Autodesk Inventor part; units mm, degrees
ref_plane "YZ Plane" through (0, 0, 0) normal (1, 0, 0) x (0, 1, 0)
ref_plane "XZ Plane" through (0, 0, 0) normal (0, 1, 0) x (-1, 0, 0)
ref_plane "XY Plane" through (0, 0, 0) normal (0, 0, 1) x (1, 0, 0)
sketch "Sketch1" plane through (0, 0, 0) normal (0, 0, 1) x (1, 0, 0)
  arc A0 (-39.344, -1.4316) -> (39.344, -1.4316) centre (0, 0) ccw
  line L0 (-39.344, -1.4316) -> (-39.3671, -1.4316)
  line L1 (-39.344, -1.4316) -> (-52.044, -1.4316)
  line L2 (39.344, -1.4316) -> (52.044, -1.4316)
  arc A1 (-46.964, -22.4724) -> (46.964, -22.4724) centre (0, 0) ccw
  line L3 (0, -52.0636) -> (0, -55.2386)
  line L4 (0, -55.2386) -> (-72.364, -55.2386)
  line L5 (0, -55.2386) -> (72.364, -55.2386)
  line L6 (-52.044, -1.4316) -> (-59.664, -1.4316)
  line L7 (52.044, -1.4316) -> (59.664, -1.4316)
  line L8 (39.344, -1.4316) -> (46.964, -1.4316)
  line L9 (46.964, -1.4316) -> (46.964, -22.4724)
  line L10 (-39.344, -1.4316) -> (-45.694, -1.4316)
  line L11 (-39.344, -1.4316) -> (-46.964, -1.4316)
  line L12 (-46.964, -1.4316) -> (-46.964, -22.4724)
  line L13 (-46.964, -7.7816) -> (-59.664, -7.7816)
  line L14 (-59.664, -7.7816) -> (-59.664, -1.4316)
  line L15 (46.964, -7.7816) -> (59.664, -7.7816)
  line L16 (59.664, -7.7816) -> (59.664, -1.4316)
  line L17 (-72.364, -55.2386) -> (-72.364, -42.5386)
  line L18 (72.364, -55.2386) -> (72.364, -42.5386)
  line L19 (-72.364, -42.5386) -> (-30.0181, -42.5386)
  line L20 (72.364, -42.5386) -> (30.0181, -42.5386)
  dimension "d0" = 78.74
  dimension "d2" = 12.7
  dimension "d3" = 12.7
  dimension "d4" = 3.175
  dimension "d5" = 7.62
  dimension "d6" = 7.62
  dimension "d7" = 7.62
  dimension "d9" = 7.62
  dimension "d10" = 6.35
  dimension "d11" = 6.35
  dimension "d14" = 12.7
  dimension "d15" = 12.7
extrude "Extrusion1" add sketch "Sketch1" along normal blind 12.7
fillet "Fillet1" radius 7.62 2 edges at (30.0181, -42.5386, 6.35) (-30.0181, -42.5386, 6.35)
fillet "Fillet2" radius 25.4 2 edges at (-46.964, -22.4724, 6.35) (46.964, -22.4724, 6.35)
sketch "Sketch2" plane through (-59.664, -1.4316, 0) normal (0, 1, 0) x (1, 0, 0)
  line L0 (0, 0) -> (0, -12.7)
  line L1 (99.0079, 0) -> (20.32, 0)
  line L2 (0, 0) -> (20.32, 0)
  circle A0 centre (7.62, -6.35) radius 4.064
  circle A1 centre (111.7079, -6.35) radius 4.064
  line L3 (119.3279, 0) -> (119.3279, -12.7)
  line L4 (-12.7, 0) -> (132.0279, 0)
  line L5 (119.3279, 0) -> (132.0279, 0)
  circle A2 centre (125.6779, -6.35) radius 4.064
  line L6 (-12.7, 0) -> (0, 0)
  circle A3 centre (-6.35, -6.35) radius 4.064
  line L7 (20.32, 0) -> (20.32, -12.7)
  line L8 (99.0079, 0) -> (99.0079, -12.7)
  point P0 (59.664, 0)
  dimension "d20" = 8.128
  dimension "d21" = 8.128
  dimension "d22" = 8.128
  dimension "d23" = 8.128
  dimension "d24" = 12.7
  dimension "d25" = 12.7
extrude "Extrusion2" cut sketch "Sketch2" against normal blind 25.4 contours A0 | A1
extrude "Extrusion3" cut sketch "Sketch2" against normal blind 76.2 contours A2 | A3
properties part number "MOTOR MOUNT REAL BOTTOM"
Design review of the part built by this model. Coordinates are the model's own, in mm. A direction names the side the tool comes from. Give positions to 0.01 mm unless a question says otherwise; leave off trailing zeros. Loops run counter-clockwise (first coordinate to the right, second up) from the corner with the lowest first, then second, coordinate; pieces in that order, holes last. Notation, with made-up numbers: M 77,-4 L 82,-4 A30 ccw 82,30 Z; hole C 46.5,61.5 d11. An arc over 180 degrees is marked long. One line per question, with ' | ' between items. Start each with the question number.
1. To check wall thickness, follow L1, parallel to X at y = -48.5, z = 6.35; L2, parallel to Y at x = 56, z = 8; L3, parallel to X at y = -5, z = 6.35. State the ranges of each line that lie inside material, in increasing order.
2. Add section C-C (z = 6.35). Give the number of separate pieces and of enclosed holes in the cut face, plus the area to 3 significant figures.
3. Add section A-A (y = -5). Write out the cut boundary in (x, z), plus the area to 3 significant figures.
4. Add section B-B (y = -13.5). Write out the cut boundary in (x, z).
5. Insertion check: P1, Ø6.5, axis at x = 52.04, z = 6.35, coming from the +Y side; P2, Ø1.9, axis at y = -5.5, z = 6, coming from the +X side; P3, Ø3, axis at x = -18.5, z = 7.5, coming from the +Y side; P4, Ø6, axis at x = 37.5, y = -32, coming from the -Z side. Each pin has a flat end and moves straight along its axis. Give the tip position at first contact, or say it passes through.
6. Add section D-D (x = 0). Write out the cut boundary in (y, z), plus the area to 3 significant figures.
7. For faces 4 (the face through (-59.664, -5, 6)), 5 (the face through (59.664, -5, 6)), 6 (the face through (61, -42.539, 6)), 7 (the face through (-46.964, -12, 6)), list the 3-axis set-ups (+Z, -Z, +X, -X, +Y, -Y) from which the entire face can be reached by the end or side of a thin tool; tool diameter is ignored.
8. The part is to be moulded in two halves that separate along X. For faces 1 (the face through (-1, -40, 12.7)), 2 (the face through (41.572, -38.296, 6.439)), 3 (the face through (-48.168, -4.562, 5.129)), say which applies: released by +X, released by -X, zero draft, split by the parting line, or undercut.
Worked out:
1) L1: x = -72.36 to -70.08, -61.95 to 61.95, 70.08 to 72.36 | L2: y = -55.24 to -42.54, -7.78 to -1.43 | L3: x = -59.66 to -56.11, -47.98 to -39.05, 39.05 to 47.98, 56.11 to 59.66
2) separate pieces: 5 | enclosed holes: 0 | area: 3,060 mm²
3) outline: M -59.66,0 L -39.05,0 L -39.05,12.7 L -59.66,12.7 Z; M 39.05,0 L 59.66,0 L 59.66,12.7 L 39.05,12.7 Z; hole C -52.04,6.35 d8.13; hole C 52.04,6.35 d8.13 | area: 420 mm²
4) outline: M -46.96,0 L -36.98,0 L -36.98,12.7 L -46.96,12.7 Z; M 36.98,0 L 46.96,0 L 46.96,12.7 L 36.98,12.7 Z
5) P1: stops at y = -42.54 | P2: stops at x = 59.66 | P3: stops at y = -33.91 | P4: stops at z = 0
6) outline: M -55.24,0 L -39.37,0 L -39.37,12.7 L -55.24,12.7 Z | area: 202 mm²
7) face 4: +Z, -Z, -X, +Y | face 5: +Z, -Z, +X, +Y | face 6: +Z, -Z, +X | face 7: +Z, -Z, -X
8) face 1: zero draft | face 2: released by +X | face 3: undercut
